CAD build for the part. Positions are in the model's coordinates, mm. Face numbers are marked on the shaded views. A direction names the side the tool comes from. Give positions to 0.01 mm unless a question says otherwise; leave off trailing zeros. Order: outer loops, then holes, each group sorted by start corner. A loop starts at its lowest first (then second) coordinate and runs counter-clockwise, first axis right, second up.
from build123d import *

# Parameters (mm, degrees)
SKETCH2_R           = 14
BOSS_EXTRUDE1_DEPTH = 4
SKETCH3_R           = 7.5
BOSS_EXTRUDE2_DEPTH = 12
SKETCH4_R           = 3.01
CUT_EXTRUDE1_DEPTH  = 17
SKETCH5_R           = 1.6
CUT_EXTRUDE2_DEPTH  = 12


with BuildPart() as part:
    # Sketch2 → Boss-Extrude1 (new body)
    with BuildSketch(Plane(origin=(0, 0, 0), x_dir=(1, 0, 0), z_dir=(0, 1, 0))):
        Circle(SKETCH2_R)
    extrude(amount=BOSS_EXTRUDE1_DEPTH)

    # Sketch3 → Boss-Extrude2 (add)
    with BuildSketch(Plane(origin=(0, 4, 0), x_dir=(1, 0, 0), z_dir=(0, 1, 0))):
        Circle(SKETCH3_R)
    extrude(amount=BOSS_EXTRUDE2_DEPTH)

    # Sketch4 → Cut-Extrude1 (cut, through all)
    with BuildSketch(Plane(origin=(0, 16, 0), x_dir=(1, 0, 0), z_dir=(0, 1, 0))):
        Circle(SKETCH4_R)
    extrude(amount=-CUT_EXTRUDE1_DEPTH, mode=Mode.SUBTRACT)

    # Sketch5 → Cut-Extrude2 (cut)
    with BuildSketch(Plane(origin=(0, 4, 0), x_dir=(1, 0, 0), z_dir=(0, 1, 0))):
        with Locations((0, -10.5)):
            Circle(SKETCH5_R)
        with Locations((9.09326674, 5.25)):
            Circle(SKETCH5_R)
        with Locations((-9.09326674, 5.25)):
            Circle(SKETCH5_R)
    extrude(amount=-CUT_EXTRUDE2_DEPTH, mode=Mode.SUBTRACT)


solid = part.part
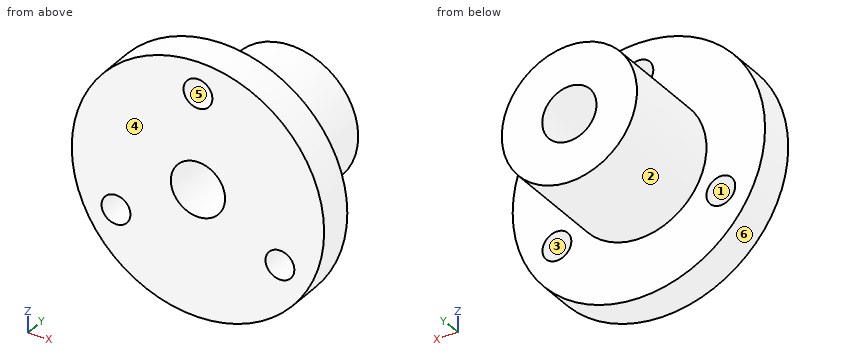
1. Saw through at C-C on x = 8.25. Give the cut face in (y, z), plus the area to 3 significant figures.
2. Saw through at B-B on x = 0. Give the cut face in (y, z).
3. Pin check, flat tips, straight feed: P1, Ø10, axis at x = -1, z = 2.5, coming from the -Y side; P2, Ø1.9, axis at x = 9.09, z = -5.25, coming from the -Y side; P3, Ø5, axis at y = 1.5, z = -7.5, coming from the -X side; P4, Ø3, axis at y = 7.5, z = -5.5, coming from the +X side. Stop position of each tip, or through.
4. 3-axis set-ups, long thin cutter, end or side, ignore diameter. For the marked faces 1 and 2: which of +Z, -Z, +X, -X, +Y, -Y reach the whole face in a straight line?
5. Mould opens along X. For the marked faces 3, 4, 5 and 6 say: released by +X, released by -X, zero draft, split by the parting line, or undercut.
6. Saw through at D-D on y = 2. Give the cut face in (x, z).
7. Saw through at A-A on z = 0. Give the cut face in (x, y).
8. Wall check: line 1 (Z direction, x = 0, y = 1.1); line 2 (X direction, y = 11.75, z = 0); line 3 (X direction, y = 2.1, z = -5.25). Give the ranges that are in metal, low to high.
Reported:
1. outline: (0, -11.31) - (4, -11.31) - (4, -6.61) - (0, -6.61) - close; (0, -3.89) - (4, -3.89) - (4, 11.31) - (0, 11.31) - close
1. area: 79.6 mm2
2. outline: (0, -14) - (4, -14) - (4, -7.5) - (16, -7.5) - (16, -3.01) - (0, -3.01) - close; (0, 3.01) - (16, 3.01) - (16, 7.5) - (4, 7.5) - (4, 8.9) - (0, 8.9) - close; (0, 12.1) - (4, 12.1) - (4, 14) - (0, 14) - close
3. P1: stops at y = 0
3. P2: passes through
3. P3: stops at x = -13.08
3. P4: stops at x = 6.34
4. face 1: +Y, -Y
4. face 2: +Y
5. face 3: undercut
5. face 4: zero draft
5. face 5: undercut
5. face 6: split by the parting line
6. outline: circle Ø28 at (0, 0); hole circle Ø3.2 at (-9.09, -5.25); hole circle Ø6.02 at (0, 0); hole circle Ø3.2 at (0, 10.5); hole circle Ø3.2 at (9.09, -5.25)
7. outline: (-14, 0) - (-3.01, 0) - (-3.01, 16) - (-7.5, 16) - (-7.5, 4) - (-14, 4) - close; (3.01, 0) - (14, 0) - (14, 4) - (7.5, 4) - (7.5, 16) - (3.01, 16) - close
8. line 1: z = -14 to -3.01, 3.01 to 8.9, 12.1 to 14
8. line 2: x = -7.5 to -3.01, 3.01 to 7.5
8. line 3: x = -12.98 to -10.69, -7.49 to 7.49, 10.69 to 12.98
